Answer from the drawing. Dimensions are ordinates in mm from the lowest x, y and z of the part. A direction names the side the tool comes from. Give positions to 0.01 mm unless a question says otherwise; leave off trailing zeros. Write each loop counter-clockwise with the first axis right and the second up, starting at its lowest first coordinate (ties: lowest second). Pieces come first, ordered by that corner, then holes.
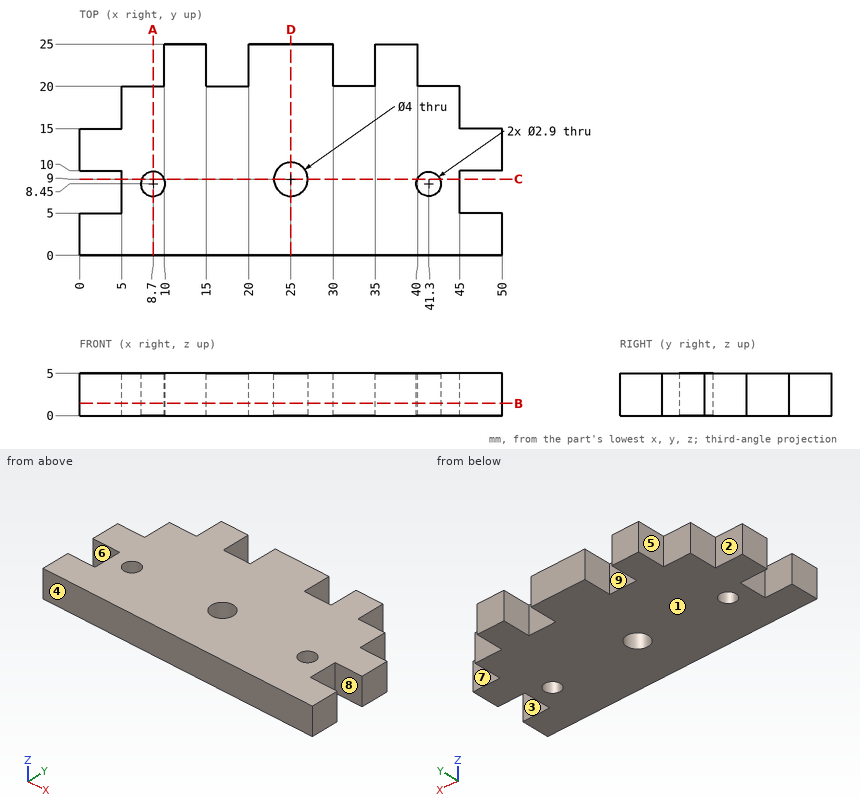
Item 1: A cutting plane is placed at C-C, the plane y = 9. Give the vertices of the cut face in (x, z), plus the area to 3 significant figures.
Conclusion:
outline: (5, 0) - (7.36, 0) - (7.36, 5) - (5, 5) - close; (10.04, 0) - (23, 0) - (23, 5) - (10.04, 5) - close; (27, 0) - (39.96, 0) - (39.96, 5) - (27, 5) - close; (42.64, 0) - (45, 0) - (45, 5) - (42.64, 5) - close
area: 153 mm2
Item 2: A cutting plane is placed at D-D, the plane x = 25. Give the vertices of the cut face in (y, z), plus the area to 3 significant figures.
Conclusion:
outline: (0, 0) - (7, 0) - (7, 5) - (0, 5) - close; (11, 0) - (25, 0) - (25, 5) - (11, 5) - close
area: 105 mm2
Item 3: A cutting plane is placed at B-B, the plane z = 1.45. Count the separate pieces of the cut face and the enclosed holes in it, plus the area to 3 significant figures.
Conclusion:
separate pieces: 1
enclosed holes: 3
area: 974 mm2
Item 4: A cutting plane is placed at A-A, the plane x = 8.7. Give the vertices of the cut face in (y, z), plus the area to 3 significant figures.
Conclusion:
outline: (0, 0) - (7, 0) - (7, 5) - (0, 5) - close; (9.9, 0) - (20, 0) - (20, 5) - (9.9, 5) - close
area: 85.5 mm2
Item 5: Determine the mould class of the marked faces 1, 2, 3 and 4 for opening direction Y: pulls with the +Y half, pulls with the -Y half, needs draft (parallel to the pull), parting line crosses it, or undercut.
Conclusion:
face 1: needs draft
face 2: pulls with the +Y half
face 3: undercut
face 4: pulls with the -Y half
Item 6: Which of the six approach directions +Z, -Z, +X, -X, +Y, -Y give full straight-line access (tool end or side, diameter ignored) to the marked faces 5, 6, 7, 8 and 9?
Conclusion:
face 5: +Z, -Z, -X, +Y
face 6: +Z, -Z, -X
face 7: +Z, -Z, +X, +Y
face 8: +Z, -Z, +X
face 9: +Z, -Z, +Y
Item 7: Each of these flat-tipped pins is pushed along its axis until it touches: P1, Ø2.5, axis at y = 22, z = 2, coming from the -X side; P2, Ø2.5, axis at y = 18, z = 2.5, coming from the +X side; P3, Ø2.5, axis at y = 17.5, z = 2, coming from the -X side. Where does it stop, or does it pass through?
Conclusion:
P1: stops at x = 10
P2: stops at x = 45
P3: stops at x = 5
Item 8: Consider probe 1 along Y at (x, z) = (41.3, 1.1); probe 2 along X at (y, z) = (8.25, 1.85); probe 3 along Y at (x, z) = (48.5, 1.9). Determine where each line is inside the solid, lowest interval first.
Conclusion:
probe 1: y = 0 to 7, 9.9 to 20
probe 2: x = 5 to 7.26, 10.14 to 23.15, 26.85 to 39.86, 42.74 to 45
probe 3: y = 0 to 5, 10 to 15
